Could you check a few things on this model? Use its own coordinates, in mm. Face numbers are marked on the shaded views. A direction names the side the tool comes from. Give positions to 0.01 mm unless a question says otherwise; leave off trailing zeros. Loops run counter-clockwise (first coordinate to the right, second up) from the corner with the lowest first, then second, coordinate; pieces in that order, holes last. Notation, with made-up numbers: (74.5, 19) -> (110.5, 19) arc R19 cw to (110.5, 27) -> close; hole circle Ø8 at (68, 65). An arc over 180 degrees is marked (long way). Write each question's results on one line, items separated by ' | '. Start each with the question number.
Q1. If we section it at A-A, the plane z = -5: List the corners of the cut face in (x, y) for me.
Q2. If I drill on line 1 along X through (y, z) = (0, 12.5); line 2 along X through (y, z) = (0, 3) (3 decimals); line 3 along Z through (x, y) = (0.5, -4.25), over which ranges is the centre line in solid material (lowest first)?
Q3. Which directions (+Z, -Z, +X, -X, +Y, -Y) give clear straight access to the entire face, cutting with the end or side of a thin tool? Please do the marked faces 1 and 2.
Q4. We'd pull the mould along Y, two halves only. Please class the marked faces 3, 4, 5 and 6: released by +Y, released by -Y, zero draft, split by the parting line, or undercut.
Q5. Will these pins go through, and if not, where does the flat tip stop? P1, Ø11.5, axis at x = 0, y = 0, coming from the -Z side; P2, Ø5, axis at y = -4, z = 20, coming from the -X side; P3, Ø5, axis at y = -3, z = -8.5, coming from the -X side; P4, Ø4, axis at x = 0, y = 0, coming from the -Z side.
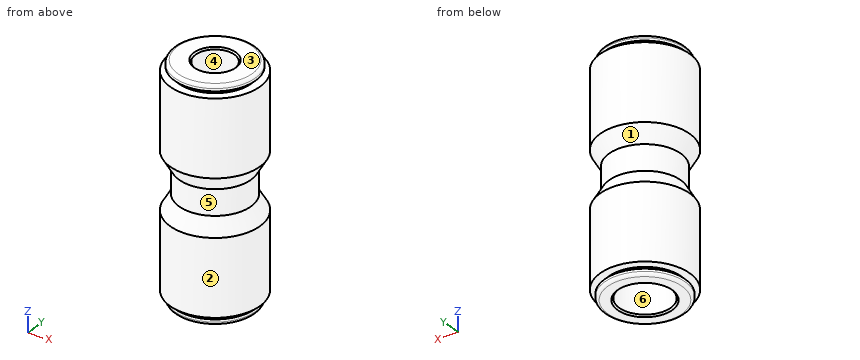
from build123d import *


with BuildPart() as part:
    # Sketch1 → Revolve1 (revolve)
    with BuildSketch(Plane(origin=(0, 0, 0), x_dir=(0, 0, -1), z_dir=(1, 0, 0)), mode=Mode.PRIVATE) as revolve1_sk:
        with BuildLine():
            Line((26.543, 9.9441), (27.178, 9.9441))
            ThreePointArc((27.178, 9.9441), (27.716815367, 9.720915367), (27.94, 9.1821))
            Line((27.94, 9.1821), (27.94, 6.731))
            Line((27.94, 6.731), (27.559, 6.35))
            Line((27.559, 6.35), (0.254, 6.35))
            Line((0.254, 6.35), (0.254, 3.175))
            Line((0.254, 3.175), (-7.112, 3.175))
            Line((-7.112, 3.175), (-7.112, 4.7625))
            Line((-7.112, 4.7625), (-27.559, 4.7625))
            Line((-27.559, 4.7625), (-27.94, 5.1435))
            Line((-27.94, 5.1435), (-27.94, 9.1821))
            ThreePointArc((-27.94, 9.1821), (-27.716815367, 9.720915367), (-27.178, 9.9441))
            Line((-27.178, 9.9441), (-26.543, 9.9441))
            Line((-26.543, 9.9441), (-26.543, 8.94969))
            Line((-26.543, 8.94969), (-25.527, 8.94969))
            Line((-25.527, 8.94969), (-25.527, 11.049))
            Line((-25.527, 11.049), (-6.931930319, 11.049))
            Line((-6.931930319, 11.049), (-3.104444444, 8.8392))
            Line((-3.104444444, 8.8392), (3.104444444, 8.8392))
            Line((3.104444444, 8.8392), (6.931930319, 11.049))
            Line((6.931930319, 11.049), (25.527, 11.049))
            Line((25.527, 11.049), (25.527, 8.94969))
            Line((25.527, 8.94969), (26.543, 8.94969))
            Line((26.543, 8.94969), (26.543, 9.9441))
        make_face()
    revolve(revolve1_sk.sketch.rotate(Axis((0, 0, 0), (0, 0, -1)), 180), axis=Axis((0, 0, 0), (0, 0, -1)))


solid = part.part
Final values:
1) outline: circle Ø19.87 at (0, 0); hole circle Ø12.7 at (0, 0)
2) line 1: x = -11.05 to -4.76, 4.76 to 11.05 | line 2: x = -8.839 to -3.175, 3.175 to 8.839 | line 3: z = -0.25 to 7.11
3) face 1: none | face 2: +Z, -Z
4) face 3: zero draft | face 4: undercut | face 5: split by the parting line | face 6: undercut
5) P1: stops at z = -0.25 | P2: stops at x = -10.95 | P3: stops at x = -11.04 | P4: passes through
